Read the model definition and answer for the solid it produces. Units are mm, in the model's axes. A direction names the side the tool comes from. Give positions to 0.01 mm unless a question says otherwise; leave off trailing zeros. Write each loop counter-clockwise with the first axis right and the second up, starting at its lowest first coordinate (ties: lowest second). Pieces come first, ordered by that corner, then holes. Notation, with made-up numbers: M 21,26 L 52,26 A31 cw 52,50 Z; hole C 89,8.25 d9. An arc over 180 degrees is marked long. Answer as CSV lines item,"result". Start each with the question number.
```python
from build123d import *

# Parameters (mm, degrees)
SKETCH1_W           = 4.980670257
SKETCH1_H           = 54.9718421
BOSS_EXTRUDE1_DEPTH = 10
SKETCH2_W           = 1.980670257
SKETCH2_H           = 15
CUT_EXTRUDE2_DEPTH  = 7
SKETCH4_W           = 1.980670257
SKETCH4_H           = 25.98592105
CUT_EXTRUDE3_DEPTH  = 7


with BuildPart() as part:
    # Sketch1 → Boss-Extrude1 (new body)
    with BuildSketch(Plane(origin=(0, 0, 0), x_dir=(1, 0, 0), z_dir=(0, 1, 0))):
        with Locations((-11.806033203, 3.043742935)):
            Rectangle(SKETCH1_W, SKETCH1_H)
    extrude(amount=BOSS_EXTRUDE1_DEPTH)

    # Sketch2 → Cut-Extrude2 (cut)
    with BuildSketch(Plane(origin=(0, 10, 0), x_dir=(1, 0, 0), z_dir=(0, 1, 0))):
        with Locations((-11.806033203, 10.543742935)):
            Rectangle(SKETCH2_W, SKETCH2_H)
    extrude(amount=-CUT_EXTRUDE2_DEPTH, mode=Mode.SUBTRACT)

    # Sketch4 → Cut-Extrude3 (cut)
    with BuildSketch(Plane.XZ):
        with Locations((-11.806033203, 9.94921759)):
            Rectangle(SKETCH4_W, SKETCH4_H)
    extrude(amount=-CUT_EXTRUDE3_DEPTH, mode=Mode.SUBTRACT)


solid = part.part
```
1. Given pin 1 (1 mm diameter, centred on x = -12, z = 8.5, fed in from -Y), flat-ended and moving along its own axis, determine where the tip first touches the part or whether it passes through.
2. Find section C-C on z = -4. Determine the outline of the cut face in (x, y), then the cut area to 3 significant figures.
3. For faces 1 (the face through (-12.796, 5, 2)), 2 (the face through (-11.8, 0, -3.4)), 3 (the face through (-12, 1, -3.044)), 4 (the face through (-12, 9, -3.044)), 5 (the face through (-9.316, 5, -3)), determine the directions among +Z, -Z, +X, -X, +Y, -Y from which every point of the face is accessible in a straight line to the end or side of a thin tool.
4. Find the intervals of material crossed by line 1 (X direction, y = 6.25, z = 13); line 2 (Z direction, x = -10.95, y = 8); line 3 (Z direction, x = -12.6, y = 5.25), in increasing order. Write a range as [from, to].
5. Determine the mould class of faces 6 (the face through (-12, 5, -30.53)), 7 (the face through (-14.296, 5, -3)), 8 (the face through (-12, 3, 22.942)) for opening direction Z: +Z half, -Z half, draft (parallel to the pull), parting line (faces both ways), or undercut.
6. Find section A-A on x = -11.75. Determine the outline of the cut face in (y, z).
7. Find section B-B on y = 6.5. Determine the outline of the cut face in (x, z), then the cut area to 3 significant figures.
8. Find section D-D on y = 9.5. Determine the outline of the cut face in (x, z), then the cut area to 3 significant figures.
Computed:
1,pin 1,"stops at y = 7"
2,outline,"M -14.3,0 L -9.32,0 L -9.32,10 L -10.82,10 L -10.82,3 L -12.8,3 L -12.8,10 L -14.3,10 Z"
2,area,"35.9 mm^2"
3,face 1,"none"
3,face 2,"+Z, -Z, +X, -X, -Y"
3,face 3,"-Y"
3,face 4,"+Y"
3,face 5,"+Z, -Z, +X, +Y, -Y"
4,line 1,"x = [-14.3, -12.8], [-10.82, -9.32]"
4,line 2,"z = [-30.53, -18.04], [-3.04, 24.44]"
4,line 3,"z = [-30.53, -18.04], [22.94, 24.44]"
5,face 6,"-Z half"
5,face 7,"draft"
5,face 8,"undercut"
6,outline,"M 0,-30.53 L 10,-30.53 L 10,-18.04 L 3,-18.04 L 3,-3.04 L 0,-3.04 Z; M 0,22.94 L 7,22.94 L 7,-3.04 L 10,-3.04 L 10,24.44 L 0,24.44 Z"
7,outline,"M -14.3,-30.53 L -9.32,-30.53 L -9.32,24.44 L -14.3,24.44 Z; hole M -12.8,-18.04 L -10.82,-18.04 L -10.82,22.94 L -12.8,22.94 Z"
7,area,"193 mm^2"
8,outline,"M -14.3,-30.53 L -9.32,-30.53 L -9.32,24.44 L -14.3,24.44 Z; hole M -12.8,-18.04 L -10.82,-18.04 L -10.82,-3.04 L -12.8,-3.04 Z"
8,area,"244 mm^2"
